Verification items for the finished model (mm, model axes). A direction names the side the tool comes from. Round coordinates to 2 decimals unless told otherwise and drop trailing zeros. Write each loop counter-clockwise with the first axis right and the second up, starting at its lowest first coordinate (ties: lowest second). Pieces come first, ordered by that corner, then holes. Notation, with made-up numbers: (24, 65) - (56, 65) arc R7 ccw to (56, 74) - close; hole circle Ø7 at (-1.75, 87.5). An arc over 180 degrees is marked (long way). Answer as a JSON object with one key per item and string values.
```python
from build123d import *

# Parameters (mm, degrees)
SKETCH1_R                                         = 31.369
BOSS_EXTRUDE1_DEPTH                               = 12.7
SKETCH2_R                                         = 19.177
CUT_EXTRUDE1_DEPTH                                = 47.144537293
CUT_EXTRUDE2_START                                = -9.525
SKETCH3_R                                         = 26.289
CUT_EXTRUDE2_DEPTH                                = 9.525
CHAMFER1_SIZE                                     = 2.54
CSK_FOR_2_FLAT_HEAD_MACHINE_SCREW_100_D           = 2.4384
CSK_FOR_2_FLAT_HEAD_MACHINE_SCREW_100_CSINK_D     = 4.3688
CSK_FOR_2_FLAT_HEAD_MACHINE_SCREW_100_CSINK_ANGLE = 82
F_4_40_TAPPED_HOLE1_D                             = 2.2606
F_4_40_TAPPED_HOLE1_DEPTH                         = 7.5946
F_4_40_TAPPED_HOLE1_CSINK_D                       = 3.175
F_4_40_TAPPED_HOLE1_CSINK_ANGLE                   = 90
F_4_40_TAPPED_HOLE1_TIP                           = 0.679152758
SKETCH12_W                                        = 12.7
SKETCH12_H                                        = 8.945423361
CUT_EXTRUDE3_DEPTH                                = 7.62
CUT_EXTRUDE4_DEPTH                                = 51.675705442
CUT_EXTRUDE4_DEPTH_BACK                           = 51.675705442
SKETCH13_R                                        = 1.1938


with BuildPart() as part:
    # Sketch1 → Boss-Extrude1 (new body)
    with BuildSketch(Plane.XY):
        Circle(SKETCH1_R)
    extrude(amount=BOSS_EXTRUDE1_DEPTH)

    # Sketch2 → Cut-Extrude1 (cut, through all)
    with BuildSketch(Plane(origin=(0, 0, 0), x_dir=(-1, 0, 0), z_dir=(0, 0, -1))):
        Circle(SKETCH2_R)
    extrude(amount=-CUT_EXTRUDE1_DEPTH, mode=Mode.SUBTRACT)

    # Sketch3 → Cut-Extrude2 (cut)
    with BuildSketch(Plane.XY.offset(12.7).offset(CUT_EXTRUDE2_START)):
        Circle(SKETCH3_R)
    extrude(amount=CUT_EXTRUDE2_DEPTH, mode=Mode.SUBTRACT)

    # Chamfer1
    chamfer1_edges = [part.edges().sort_by_distance(p)[0] for p in [
        (-31.369, 0, 12.7),
    ]]
    chamfer(chamfer1_edges, length=CHAMFER1_SIZE)

    # CSK for #2 Flat Head Machine Screw (100)1 (through all)
    with Locations(Plane.XY.offset(3.175)):
        with Locations((-15.367, -15.367), (-15.367, 15.367), (15.367, 15.367), (15.367, -15.367)):
            CounterSinkHole(CSK_FOR_2_FLAT_HEAD_MACHINE_SCREW_100_D / 2, CSK_FOR_2_FLAT_HEAD_MACHINE_SCREW_100_CSINK_D / 2, counter_sink_angle=CSK_FOR_2_FLAT_HEAD_MACHINE_SCREW_100_CSINK_ANGLE)

    # #4-40 Tapped Hole1
    with Locations(Plane(origin=(0, 0, 0), x_dir=(-1, 0, 0), z_dir=(0, 0, -1))):
        with Locations((-20.32, 20.32), (20.32, 20.32), (20.32, -20.32), (-20.32, -20.32)):
            CounterSinkHole(F_4_40_TAPPED_HOLE1_D / 2, F_4_40_TAPPED_HOLE1_CSINK_D / 2, depth=F_4_40_TAPPED_HOLE1_DEPTH, counter_sink_angle=F_4_40_TAPPED_HOLE1_CSINK_ANGLE)
            with Locations((0, 0, -(F_4_40_TAPPED_HOLE1_DEPTH + F_4_40_TAPPED_HOLE1_TIP / 2))):  # 118° drill point
                Cone(0, F_4_40_TAPPED_HOLE1_D / 2, F_4_40_TAPPED_HOLE1_TIP, mode=Mode.SUBTRACT)

    # Sketch12 → Cut-Extrude3 (cut)
    with BuildSketch(Plane.XY.offset(12.7)):
        with Locations((0, 26.89628832)):
            Rectangle(SKETCH12_W, SKETCH12_H)
    extrude(amount=-CUT_EXTRUDE3_DEPTH, mode=Mode.SUBTRACT)

    # Sketch13 → Cut-Extrude4 (cut, two sides: drawn at the far end of the back side and taken through both)
    with BuildSketch(Plane(origin=(-6.35, 0, 0), x_dir=(0, 0, -1), z_dir=(1, 0, 0)).offset(-CUT_EXTRUDE4_DEPTH_BACK)):
        with Locations(Location((-7.62, 27.925564792, 0), (0, 0, 90))):
            Circle(SKETCH13_R)
    extrude(amount=CUT_EXTRUDE4_DEPTH + CUT_EXTRUDE4_DEPTH_BACK, mode=Mode.SUBTRACT)


solid = part.part
```
1. Material ranges on probe 1 along X at (y, z) = (-20.32, 6); probe 2 along Z at (x, y) = (24.5, -2) (3 decimals), recorded low to high. Write a range as from..to.
Completed:
{"probe 1": "x = -23.9..-21.45, -19.19..-16.68, 16.68..19.19, 21.45..23.9", "probe 2": "z = 0..3.175"}
2. Go/stop test with flat-tipped pins: pin 1 (2.5 mm diameter, centred on y = 27.93, z = 7.62, fed in from +X); pin 2 (1.6 mm diameter, centred on y = 27, z = 9.5, fed in from -X); pin 3 (3 mm diameter, centred on x = -15.367, y = -15.367, fed in from +Z). Record where each tip stops, or that it passes through.
Completed:
{"pin 1": "stops at x = 16.5", "pin 2": "stops at x = -17.25", "pin 3": "stops at z = 2.39"}
3. Mould release check, pull along Y, two halves, no side actions. Record for faces 5 (the face through (15.218, -11.669, 1.565)), 6 (the face through (-1.19, -28.928, 12.577)), 7 (the face through (-7, -26, 12.7)), 8 (the face through (-20, 20, 8)): released by +Y, released by -Y, zero draft, split by the parting line, or undercut.
Completed:
{"face 5": "undercut", "face 6": "split by the parting line", "face 7": "zero draft", "face 8": "undercut"}
4. Access from +Z, -Z, +X, -X, +Y, -Y to the whole of each face (thin tool, end or side, straight path). Record for faces 1 (the face through (-5.699, -25.664, 7.871)), 2 (the face through (-14.4, -16.11, 1.02)), 3 (the face through (19.423, 19.632, 4.076)), 4 (the face through (-6.35, 28, 9)).
Completed:
{"face 1": "+Z", "face 2": "+Z, -Z", "face 3": "-Z", "face 4": "+Z, +Y"}
5. Cross-section at A-A (y = 0). Record the boundary of the cut face in (x, z) (3 decimals).
Completed:
{"outline": "(-31.369, 0) - (-19.177, 0) - (-19.177, 3.175) - (-26.289, 3.175) - (-26.289, 12.7) - (-28.829, 12.7) - (-31.369, 10.16) - close; (19.177, 0) - (31.369, 0) - (31.369, 10.16) - (28.829, 12.7) - (26.289, 12.7) - (26.289, 3.175) - (19.177, 3.175) - close"}
6. Cross-section at B-B (z = 11.5). Record the boundary of the cut face in (x, y), plus the area to 3 significant figures.
Completed:
{"outline": "(-6.35, 25.51) - (-6.35, 29.35) arc R30.03 ccw (long way) to (6.35, 29.35) - (6.35, 25.51) arc R26.29 cw (long way) to start", "area": "614 mm^2"}
